```python
from build123d import *
from OCP.BRepFilletAPI import BRepFilletAPI_MakeChamfer

# Parameters (mm, degrees)
SKETCH1_W                            = 9.5
SKETCH1_H                            = 55
BOSS_EXTRUDE1_REACH                  = 497.037
BOSS_EXTRUDE1_END_RADIUS             = 20
SKETCH2_R                            = 15.5
SKETCH2_R_2                          = 12.65
BOSS_EXTRUDE2_REACH                  = 497.037
BOSS_EXTRUDE2_END_RADIUS             = 20
SKETCH3_R                            = 15.5
SKETCH3_R_2                          = 12.65
SKETCH9_W                            = 200
SKETCH9_H                            = 33.234380704
CUT_EXTRUDE2_DEPTH                   = 198.5
SKETCH8_R                            = 18
BOSS_EXTRUDE3_DEPTH                  = 15
CHAMFER1_SIZE                        = 1
CHAMFER2_SIZE                        = 1
CHAMFER2_SIZE2                       = 0.883191486
BOSS_EXTRUDE5_REACH                  = 511.879
BOSS_EXTRUDE5_END_RADIUS             = 15.5
SKETCH13_W                           = 60
SKETCH13_H                           = 31
BOSS_EXTRUDE5_DIRECTION_2_REACH      = 511.879
BOSS_EXTRUDE5_DIRECTION_2_END_RADIUS = 15.5
CHAMFER4_SIZE                        = 1
SKETCH19_R                           = 5
BOSS_EXTRUDE7_DEPTH                  = 10


with BuildPart() as part:
    # Sketch1 → Revolve1 (revolve)
    with BuildSketch(Plane(origin=(0, 0, 0), x_dir=(1, 0, 0), z_dir=(0, 1, 0)), mode=Mode.PRIVATE) as revolve1_sk:
        with Locations((-4.75, 129.48)):
            Rectangle(SKETCH1_W, SKETCH1_H)
        with Locations((-4.75, -129.48)):
            Rectangle(SKETCH1_W, SKETCH1_H)
    revolve(revolve1_sk.sketch.rotate(Axis((10.5, 0, -101.98), (0, 0, -1)), 180), axis=Axis((10.5, 0, -101.98), (0, 0, -1)))

    # Boss-Extrude1: up to this cylinder (the profile starts outside it)
    boss_extrude1_end = Plane(origin=(10.5, 0, -44.652226), z_dir=(0, 0, 1)) * Cylinder(BOSS_EXTRUDE1_END_RADIUS, 1035.074, mode=Mode.PRIVATE)
    # Sketch2 → Boss-Extrude1 (add, up to the surface)
    with BuildSketch(Plane(origin=(-427.43, 0, -30), x_dir=(0.2315607356536785, 0, 0.9728204488514453), z_dir=(-0.9728204488514451, 0, 0.23156073565367846)), mode=Mode.PRIVATE) as boss_extrude1_sk1:
        Circle(SKETCH2_R)
        Circle(SKETCH2_R_2, mode=Mode.SUBTRACT)
    boss_extrude1_tool1 = extrude(boss_extrude1_sk1.sketch, amount=-BOSS_EXTRUDE1_REACH, mode=Mode.PRIVATE) - boss_extrude1_end
    add(boss_extrude1_tool1.solids().sort_by_distance((-430.917674, 0, -44.652226))[0])

    # Boss-Extrude2: up to this cylinder (the profile starts outside it)
    boss_extrude2_end = Plane(origin=(10.5, 0, 15.347774), z_dir=(0, 0, 1)) * Cylinder(BOSS_EXTRUDE2_END_RADIUS, 1035.074, mode=Mode.PRIVATE)
    # Sketch3 → Boss-Extrude2 (add, up to the surface)
    with BuildSketch(Plane(origin=(-427.43, 0, 30), x_dir=(-0.23156073565367818, 0, 0.9728204488514453), z_dir=(-0.9728204488514453, 0, -0.23156073565367818)), mode=Mode.PRIVATE) as boss_extrude2_sk1:
        Circle(SKETCH3_R)
        Circle(SKETCH3_R_2, mode=Mode.SUBTRACT)
    boss_extrude2_tool1 = extrude(boss_extrude2_sk1.sketch, amount=-BOSS_EXTRUDE2_REACH, mode=Mode.PRIVATE) - boss_extrude2_end
    add(boss_extrude2_tool1.solids().sort_by_distance((-423.942326, 0, 15.347774))[0])

    # Sketch9 → Cut-Extrude2 (cut, symmetric)
    with BuildSketch(Plane(origin=(-377.430188161, -137.373354004, 0), x_dir=(0, 0, 1), z_dir=(-0.9396926207859128, -0.34202014332565694, 0))):
        with Locations((0, 162.806860214)):
            Rectangle(SKETCH9_W, SKETCH9_H)
    extrude(amount=CUT_EXTRUDE2_DEPTH, both=True, mode=Mode.SUBTRACT)

    # Sketch8 → Boss-Extrude3 (add)
    with BuildSketch(Plane(origin=(-45.934180208, 126.203122901, 0), x_dir=(0, 0, -1), z_dir=(-0.34202014332565694, 0.9396926207859128, 1.048381213421869e-15))):
        with BuildLine():
            Line((-58.125498382, 358.322816903), (58.125498382, 358.322816903))
            Line((58.125498382, 358.322816903), (49.490055464, 418.322816903))
            ThreePointArc((49.490055464, 418.322816903), (0, 461.200007753), (-49.490055464, 418.322816903))
            Line((-49.490055464, 418.322816903), (-58.125498382, 358.322816903))
        make_face()
        with Locations(Location((0, 419.652816903, 0), (0, 0, 90))):
            Circle(SKETCH8_R, mode=Mode.SUBTRACT)
    extrude(amount=BOSS_EXTRUDE3_DEPTH)

    # Chamfer1
    chamfer1_edges = [part.edges().sort_by_distance(p)[0] for p in [
        (-9.5, 0, -156.98),
        (-9.5, 0, -101.98),
        (-9.5, 0, 101.98),
        (-9.5, 0, 156.98),
    ]]
    chamfer(chamfer1_edges, length=CHAMFER1_SIZE)

    # Chamfer2: one chamfer whose edges measure the first distance from different faces: ONE call of the kernel's chamfer builder (chamfer() names one face for all edges)
    chamfer2_edges_1 = [part.edges().sort_by_distance(p)[0] for p in [
        (-385.212638185, 10.697196363, 58.125498382),
    ]]
    chamfer2_side_1 = [part.faces().sort_by_distance(p)[0] for p in [
        (-413.403416809, 0.436592064, 53.807776923),
    ]]
    chamfer2_edges_2 = [part.edges().sort_by_distance(p)[0] for p in [
        (-385.212638185, 10.697196363, -58.125498382),
    ]]
    chamfer2_side_2 = [part.faces().sort_by_distance(p)[0] for p in [
        (-385.604654849, 11.774253296, 0),
    ]]
    chamfer2_edges_3 = [part.edges().sort_by_distance(p)[0] for p in [
        (-387.77778926, 17.744891019, 0),
        (-415.968567884, 7.48428672, 53.807776923),
        (-415.968567884, 7.48428672, -53.807776923),
        (-484.450726349, -17.44118054, 0),
        (-382.64748711, 3.649501708, 57.135102558),
        (-410.838265734, -6.611102592, 53.807776923),
        (-410.838265734, -6.611102592, -53.807776923),
        (-479.320424199, -31.536569852, 0),
        (-382.64748711, 3.649501708, -57.135102558),
    ]]
    chamfer2 = BRepFilletAPI_MakeChamfer(part.part.solid().wrapped)
    for e in chamfer2_edges_1:
        chamfer2.Add(CHAMFER2_SIZE, CHAMFER2_SIZE2, e.wrapped, chamfer2_side_1[0].wrapped)  # the first distance lies on this face
    for e in chamfer2_edges_2:
        chamfer2.Add(CHAMFER2_SIZE, CHAMFER2_SIZE2, e.wrapped, chamfer2_side_2[0].wrapped)  # the first distance lies on this face
    for e in chamfer2_edges_3:
        chamfer2.Add(CHAMFER2_SIZE, e.wrapped)
    add(Compound.cast(chamfer2.Shape()), mode=Mode.REPLACE)

    # Boss-Extrude5: up to this cylinder (the profile starts outside it)
    boss_extrude5_end = Plane(origin=(-326.943046764, 0, 53.918938836), z_dir=(-0.9728204488514453, 0, -0.2315607356536782)) * Cylinder(BOSS_EXTRUDE5_END_RADIUS, 1055.758, mode=Mode.PRIVATE)
    # Sketch13 → Boss-Extrude5 (add, up to the surface)
    with BuildSketch(Plane.XY, mode=Mode.PRIVATE) as boss_extrude5_sk1:
        with Locations((-314.108706206, 0)):
            Rectangle(SKETCH13_W, SKETCH13_H)
    boss_extrude5_tool1 = extrude(boss_extrude5_sk1.sketch, amount=BOSS_EXTRUDE5_REACH, mode=Mode.PRIVATE) - boss_extrude5_end
    add(boss_extrude5_tool1.solids().sort_by_distance((-314.108706, 0, 0))[0])

    # Boss-Extrude5 direction 2: up to this cylinder (the profile starts outside it)
    boss_extrude5_direction_2_end = Plane(origin=(-326.943046764, 0, -53.918938836), z_dir=(-0.9728204488514453, 0, 0.2315607356536785)) * Cylinder(BOSS_EXTRUDE5_DIRECTION_2_END_RADIUS, 1055.758, mode=Mode.PRIVATE)
    # Sketch13 → Boss-Extrude5 direction 2 (add, up to the surface)
    with BuildSketch(Plane.XY, mode=Mode.PRIVATE) as boss_extrude5_direction_2_sk1:
        with Locations((-314.108706206, 0)):
            Rectangle(SKETCH13_W, SKETCH13_H)
    boss_extrude5_direction_2_tool1 = extrude(boss_extrude5_direction_2_sk1.sketch, amount=-BOSS_EXTRUDE5_DIRECTION_2_REACH, mode=Mode.PRIVATE) - boss_extrude5_direction_2_end
    add(boss_extrude5_direction_2_tool1.solids().sort_by_distance((-314.108706, 0, 0))[0])

    # Chamfer4
    chamfer4_edges = [part.edges().sort_by_distance(p)[0] for p in [
        (-427.12856728, -15.445240802, -28.733637145),
        (-427.12856728, -15.445240802, 28.733637145),
    ]]
    chamfer(chamfer4_edges, length=CHAMFER4_SIZE)

    # Sketch19 → Boss-Extrude7 (add)
    with BuildSketch(Plane.XY.offset(15)):
        with BuildLine():
            Line((-334.108706206, -15.5), (-334.108706206, -45.5))
            ThreePointArc((-334.108706206, -45.5), (-314.108706206, -65.5), (-294.108706206, -45.5))
            Line((-294.108706206, -45.5), (-294.108706206, -15.5))
            Line((-294.108706206, -15.5), (-334.108706206, -15.5))
        make_face()
        with Locations((-314.108706206, -45.5)):
            Circle(SKETCH19_R, mode=Mode.SUBTRACT)
    boss_extrude7 = extrude(amount=BOSS_EXTRUDE7_DEPTH)

    # Mirror2: Boss-Extrude7 across plane
    add(boss_extrude7.mirror(Plane.XY))


solid = part.part
```
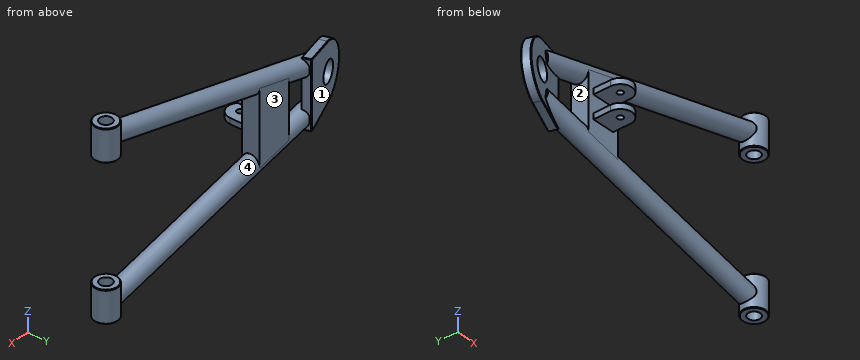
CAD build for the part. Positions are in the model's coordinates, mm. Face numbers are marked on the shaded views. A direction names the side the tool comes from. Coordinates: 2 decimals unless noted, no trailing zeros. Loops run counter-clockwise (first coordinate to the right, second up) from the corner with the lowest first, then second, coordinate; pieces in that order, holes last. Notation, with made-up numbers: (1, 0.25) - (44, 0.25) arc R10 cw to (44, 12.25) - close; hole circle Ø1 at (46.25, -31). An arc over 180 degrees is marked (long way). Use CSV: the item, a comma, the result in double quotes. Start each with the question number.
Q1. Cut at B-B, the plane z = 126. State how many separate pieces and enclosed holes the cut face has, then the cut area to 3 significant figures.
Q2. Probe probe 1 along Y at (x, z) = (10.5, -119.5); probe 2 along X at (y, z) = (-45, 22); probe 3 along Z at (x, y) = (-202, 2). List the from-to ranges inside material, lowest first. Write a range as from..to.
Q3. Two-plate mould, pull along Z, no slides. Class the marked faces 1 and 2: +Z half, -Z half, draft (parallel to the pull), parting line (faces both ways), or undercut.
Q4. Cut at A-A, the plane x = 10.5. List the corners of the cut face in (y, z).
Q5. Drop flat-ended pins along their axis: P1, Ø11, axis at y = -33, z = -20, coming from the -X side; P2, Ø12, axis at x = -317, y = -36, coming from the -Z side; P3, Ø5, axis at y = -30.5, z = -20.5, coming from the +X side. Give the stop position or say it passes through.
Q6. 3-axis set-ups, long thin cutter, end or side, ignore diameter. For the marked faces 3 and 4: which of +Z, -Z, +X, -X, +Y, -Y reach the whole face in a straight line?
Here are the results:
1,separate pieces,"1"
1,enclosed holes,"2"
1,area,"1,570 mm2"
2,probe 1,"-20..-10.5, 10.5..20"
2,probe 2,"-334.11..-319.08, -309.13..-294.11"
2,probe 3,"-99.46..-96.5, -70.82..-67.86, 67.86..70.82, 96.5..99.46"
3,face 1,"draft"
3,face 2,"undercut"
4,outline,"(-20, -155.98) - (-19, -156.98) - (-10.5, -156.98) - (-10.5, -101.98) - (-19, -101.98) - (-20, -102.98) - close; (-20, 102.98) - (-19, 101.98) - (-10.5, 101.98) - (-10.5, 156.98) - (-19, 156.98) - (-20, 155.98) - close; (10.5, -156.98) - (19, -156.98) - (20, -155.98) - (20, -102.98) - (19, -101.98) - (10.5, -101.98) - close; (10.5, 101.98) - (19, 101.98) - (20, 102.98) - (20, 155.98) - (19, 156.98) - (10.5, 156.98) - close"
5,P1,"x = -477.37"
5,P2,"z = -25"
5,P3,"x = -294.11"
6,face 3,"+Z, -Z, +X, +Y"
6,face 4,"none"
